```python
from build123d import *

# Parameters (mm, degrees)
ESQUISSE1_R             = 5.9
BOSS_EXTRU_1_DEPTH      = 9
ESQUISSE2_R             = 1.25
ENL_V_MAT_EXTRU_1_DEPTH = 3
ESQUISSE3_R             = 0.4
BOSS_EXTRU_2_DEPTH      = 3


with BuildPart() as part:
    # Esquisse1 → Boss.-Extru.1 (new body)
    with BuildSketch(Plane(origin=(0, 0, 0), x_dir=(1, 0, 0), z_dir=(0, 1, 0))):
        Circle(ESQUISSE1_R)
    extrude(amount=BOSS_EXTRU_1_DEPTH)

    # Esquisse2 → Enlèv. mat.-Extru.1 (cut)
    with BuildSketch(Plane(origin=(0, 9, 0), x_dir=(1, 0, 0), z_dir=(0, 1, 0))):
        Circle(ESQUISSE2_R)
    extrude(amount=-ENL_V_MAT_EXTRU_1_DEPTH, mode=Mode.SUBTRACT)

    # Esquisse3 → Boss.-Extru.2 (add)
    with BuildSketch(Plane.XZ):
        with Locations((3.75, 0)):
            Circle(ESQUISSE3_R)
        with Locations((-3.75, 0)):
            Circle(ESQUISSE3_R)
    extrude(amount=BOSS_EXTRU_2_DEPTH)


solid = part.part
```
Model file for the job. Use its own axes, mm. Coordinates: 2 decimals unless noted, no trailing zeros. Order: outer loops, then holes, each group sorted by start corner. A loop starts at its lowest first (then second) coordinate and runs counter-clockwise, first axis right, second up. Notation, with made-up numbers: (26, -16.75) - (52, -16.75) arc R18 cw to (52, 6.25) - close; hole circle Ø8 at (19.5, 84). An arc over 180 degrees is marked (long way). Return JSON: item names as keys, results as strings. Group by question number.
1) Mould opens along Z. For faces 1 (the flat face through (0, 6, 0)), 2 (the cylindrical face through (-5.894, 4.437, -0.259)), 3 (the flat face through (-0.1, 9, -1.4)), 4 (the cylindrical face through (-0.27, 7.52, 1.22)) say: released by +Z, released by -Z, zero draft, split by the parting line, or undercut.
2) Flat gauge pins, fed straight in: P1, Ø2, axis at x = 0, z = 0, coming from the -Y side; P2, Ø1.2, axis at x = 0, z = 0, coming from the +Y side; P3, Ø1, axis at y = 6, z = 1, coming from the +X side. Where does each tip first touch, or does it go through?
3) Saw through at A-A, the plane x = 0. Write the cut outline in (y, z), plus the area to 3 significant figures.
4) Probe line 1 (X direction, y = 7.6, z = 0); line 2 (Y direction, x = -2, z = -3). List the from-to ranges inside material, lowest first. Write a range as from..to.
5) Saw through at C-C, the plane y = -1.75. Write the cut outline in (x, z).
6) Saw through at B-B, the plane z = 0. Write the cut outline in (x, y).
7) Saw through at D-D, the plane y = 4.25. Write the cut outline in (x, z).
Values found:
{
 "1": {"face 1": "undercut", "face 2": "split by the parting line", "face 3": "zero draft", "face 4": "undercut"},
 "2": {"P1": "stops at y = 0", "P2": "stops at y = 6", "P3": "stops at x = 5.88"},
 "3": {"outline": "(0, -5.9) - (9, -5.9) - (9, -1.25) - (6, -1.25) - (6, 1.25) - (9, 1.25) - (9, 5.9) - (0, 5.9) - close", "area": "98.7 mm²"},
 "4": {"line 1": "x = -5.9..-1.25, 1.25..5.9", "line 2": "y = 0..9"},
 "5": {"outline": "circle Ø0.8 at (-3.75, 0); circle Ø0.8 at (3.75, 0)"},
 "6": {"outline": "(-5.9, 0) - (-4.15, 0) - (-4.15, -3) - (-3.35, -3) - (-3.35, 0) - (3.35, 0) - (3.35, -3) - (4.15, -3) - (4.15, 0) - (5.9, 0) - (5.9, 9) - (1.25, 9) - (1.25, 6) - (-1.25, 6) - (-1.25, 9) - (-5.9, 9) - close"},
 "7": {"outline": "circle Ø11.8 at (0, 0)"}
}
